Part model, mm, in its own coordinate system. Face numbers are marked on the shaded views. A direction names the side the tool comes from. Give positions to 0.01 mm unless a question says otherwise; leave off trailing zeros. Write each loop counter-clockwise with the first axis right and the second up, starting at its lowest first coordinate (ties: lowest second). Pieces come first, ordered by that corner, then holes. Notation, with made-up numbers: M 86,9 L 122,9 A26 cw 122,26 Z; hole C -33,67.5 d11. An arc over 180 degrees is marked long. Answer as CSV lines item,"result". Start each with the question number.
Item 1: Band-saw the part on B-B, the plane z = 19.5. List the corners of the cut face in (x, y), then the cut area to 3 significant figures.
Item 2: Band-saw the part on C-C, the plane y = 5. List the corners of the cut face in (x, z).
Item 3: Pin check, flat tips, straight feed: pin 1 (1 mm diameter, centred on y = -5.5, z = 17.5, fed in from -X); pin 2 (6 mm diameter, centred on y = -5.5, z = 17.5, fed in from +X); pin 3 (8 mm diameter, centred on x = 18, y = -2, fed in from +Z). Stop position of each tip, or through.
Item 4: Wall check: L1, parallel to Z at x = 21.25, y = -2.75. Give the ranges that are in metal, low to high. Write a range as from..to.
Item 5: Band-saw the part on A-A, the plane y = 0. List the corners of the cut face in (x, z), then the cut area to 3 significant figures.
Item 6: Band-saw the part on D-D, the plane x = 8.75. List the corners of the cut face in (y, z), then the cut area to 3 significant figures.
Item 7: 3-axis set-ups, long thin cutter, end or side, ignore diameter. For the marked faces 4 and 5: which of +Z, -Z, +X, -X, +Y, -Y reach the whole face in a straight line?
Item 8: Two-plate mould, pull along Z, no slides. Class the marked faces 1, 2 and 3: +Z half, -Z half, draft (parallel to the pull), parting line (faces both ways), or undercut.
from build123d import *

# Parameters (mm, degrees)
EXTRUDE_THIN1_DEPTH     = 8.001
CUT_EXTRUDE1_DEPTH      = 22.0058
CUT_EXTRUDE1_DEPTH_BACK = 3.0066
SKETCH7_R               = 2.4
CUT_EXTRUDE3_DEPTH      = 3.0066
CUT_EXTRUDE2_DEPTH      = 22.0058
CUT_EXTRUDE2_DEPTH_BACK = 3.0066
SKETCH8_R               = 2.4
CUT_EXTRUDE4_DEPTH      = 3.0066


with BuildPart() as part:
    # Sketch4 → Extrude-Thin1 (new body, symmetric)
    with BuildSketch(Plane(origin=(0, 0, 0), x_dir=(1, 0, 0), z_dir=(0, 1, 0))):
        with BuildLine():
            Line((23.0124, 0), (2.80924, 0))
            ThreePointArc((2.80924, 0), (0.822807346, -0.822807346), (0, -2.80924))
            Line((0, -2.80924), (0, -23.0124))
            Line((0, -23.0124), (2.0066, -23.0124))
            Line((2.0066, -23.0124), (2.0066, -2.80924))
            ThreePointArc((2.0066, -2.80924), (2.241687813, -2.241687813), (2.80924, -2.0066))
            Line((2.80924, -2.0066), (23.0124, -2.0066))
            Line((23.0124, -2.0066), (23.0124, 0))
        make_face()
    extrude(amount=EXTRUDE_THIN1_DEPTH, both=True)

    # Sketch5 → Cut-Extrude1 (cut, two sides)
    with BuildSketch(Plane(origin=(2.0066, 0, 0), x_dir=(0, 0, -1), z_dir=(1, 0, 0))) as cut_extrude1_sk:
        with BuildLine():
            Line((22.211753172, 52.125940831), (-19.812, 8.001))
            ThreePointArc((-19.812, 8.001), (-23.0124, 0), (-19.812, -8.001))
            Line((-19.812, -8.001), (22.211753172, -52.125940831))
            Line((22.211753172, -52.125940831), (-99.657131027, -52.125940831))
            Line((-99.657131027, -52.125940831), (-99.657131027, 52.125940831))
            Line((-99.657131027, 52.125940831), (22.211753172, 52.125940831))
        make_face()
    extrude(amount=CUT_EXTRUDE1_DEPTH, mode=Mode.SUBTRACT)
    extrude(cut_extrude1_sk.sketch, amount=-CUT_EXTRUDE1_DEPTH_BACK, mode=Mode.SUBTRACT)

    # Sketch7 → Cut-Extrude3 (cut, through all)
    with BuildSketch(Plane(origin=(2.0066, 0, 0), x_dir=(0, 0, -1), z_dir=(1, 0, 0))):
        with Locations((-14.0124, 0)):
            Circle(SKETCH7_R)
    extrude(amount=-CUT_EXTRUDE3_DEPTH, mode=Mode.SUBTRACT)

    # Sketch6 → Cut-Extrude2 (cut, two sides)
    with BuildSketch(Plane.XY.offset(2.0066)) as cut_extrude2_sk:
        with BuildLine():
            Line((-22.211753172, -52.125940831), (19.812, -8.001))
            ThreePointArc((19.812, -8.001), (23.0124, 0), (19.812, 8.001))
            Line((19.812, 8.001), (-22.211753172, 52.125940831))
            Line((-22.211753172, 52.125940831), (99.657131027, 52.125940831))
            Line((99.657131027, 52.125940831), (99.657131027, -52.125940831))
            Line((99.657131027, -52.125940831), (-22.211753172, -52.125940831))
        make_face()
    extrude(amount=CUT_EXTRUDE2_DEPTH, mode=Mode.SUBTRACT)
    extrude(cut_extrude2_sk.sketch, amount=-CUT_EXTRUDE2_DEPTH_BACK, mode=Mode.SUBTRACT)

    # Sketch8 → Cut-Extrude4 (cut, through all)
    with BuildSketch(Plane.XY.offset(2.0066)):
        with Locations((12.4124, 0)):
            Circle(SKETCH8_R)
    extrude(amount=-CUT_EXTRUDE4_DEPTH, mode=Mode.SUBTRACT)


solid = part.part
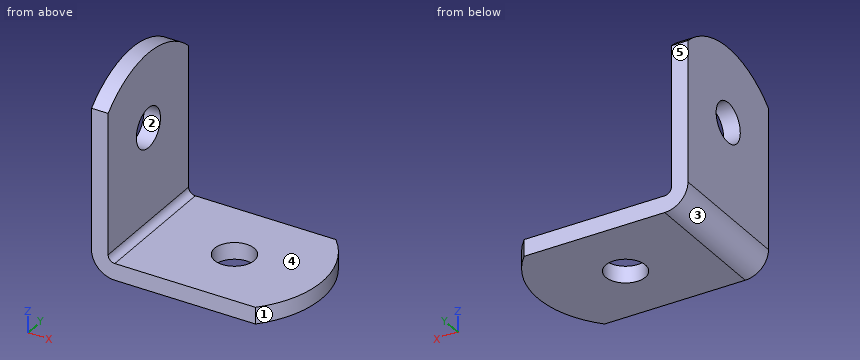
Output:
1,outline,"M 0,-8 L 2.01,-8 L 2.01,8 L 0,8 Z"
1,area,"32.1 mm²"
2,outline,"M 0,2.81 A2.81 ccw 2.81,0 L 21.88,0 L 21.88,2.01 L 2.81,2.01 A0.8 cw 2.01,2.81 L 2.01,21.88 L 0,21.88 Z"
3,pin 1,"x = 0"
3,pin 2,"x = 2.01"
3,pin 3,"z = 2.01"
4,L1,"0..2.01"
5,outline,"M 0,2.81 A2.81 ccw 2.81,0 L 10.01,0 L 10.01,2.01 L 2.81,2.01 A0.8 cw 2.01,2.81 L 2.01,11.61 L 0,11.61 Z; M 0,16.41 L 2.01,16.41 L 2.01,23.01 L 0,23.01 Z; M 14.81,0 L 23.01,0 L 23.01,2.01 L 14.81,2.01 Z"
5,area,"67.5 mm²"
6,outline,"M -8,0 L 8,0 L 8,2.01 L -8,2.01 Z"
6,area,"32.1 mm²"
7,face 4,"+Z, +X, +Y, -Y"
7,face 5,"+Z, -Z, +X, -X, +Y"
8,face 1,"draft"
8,face 2,"undercut"
8,face 3,"-Z half"
